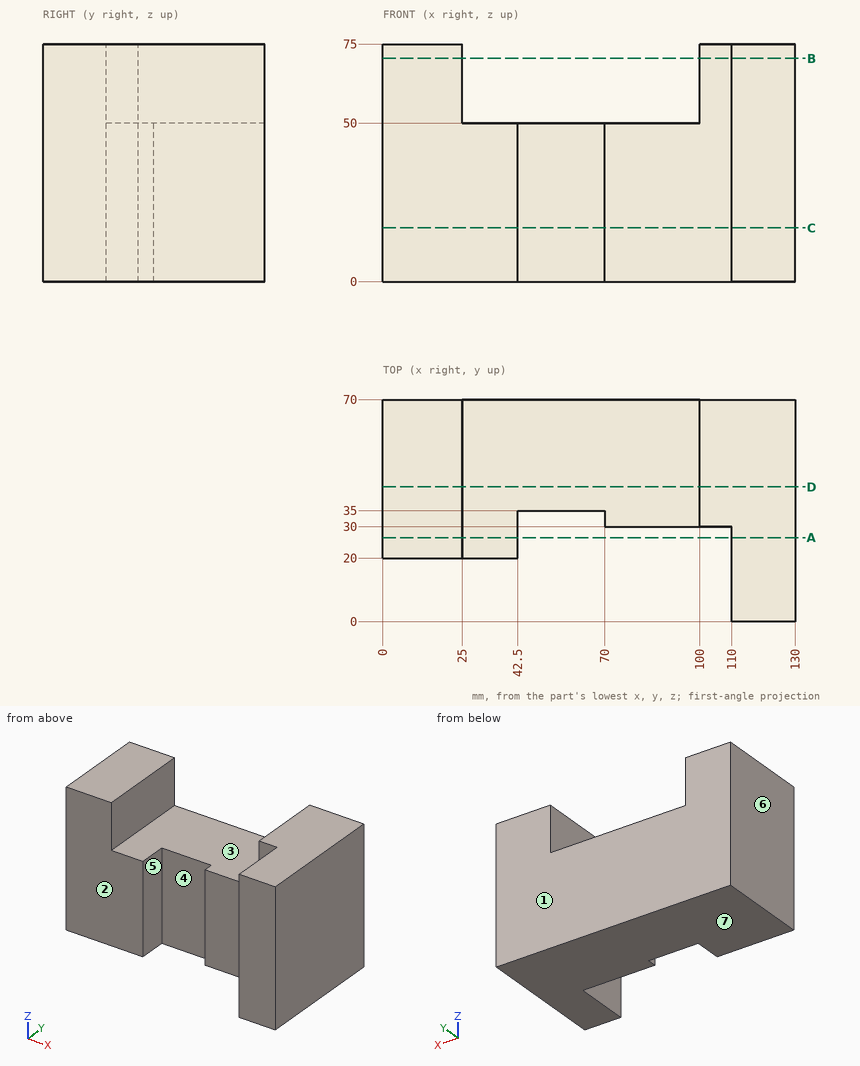
Could you check a few things on this drawing? It's one solid part, dimensions in mm from its lowest x, y, z. A direction names the side the tool comes from. Give positions to 0.01 mm unless a question says otherwise; leave off trailing zeros. Order: outer loops, then holes, each group sorted by start corner. A loop starts at its lowest first (then second) coordinate and runs counter-clockwise, first axis right, second up. Notation, with made-up numbers: M -0.75,60.5 L 51.25,60.5 A22 cw 51.25,84.5 Z; hole C 12.5,-11.75 d8. An arc over 180 degrees is marked long. Use one line per item in the form item = value. Start each with the question number.
Item 1: If we section it at B-B (z = 70.5): Write out the boundary of the cut face in (x, y).
Item 2: We'd pull the mould along X, two halves only. Please class the marked faces 5, 6 and 7: +X half, -X half, draft (parallel to the pull), parting line (faces both ways), or undercut.
Item 3: If we section it at C-C (z = 17): Write out the boundary of the cut face in (x, y), then the cut area to 3 significant figures.
Item 4: If we section it at A-A (y = 26.5): Write out the boundary of the cut face in (x, z), then the cut area to 3 significant figures.
Item 5: For the marked faces 1, 2, 3 and 4, which set-ups out of +Z, -Z, +X, -X, +Y, -Y let a thin tool reach every point of the face, with its end or its side?
Item 6: If I drill on line 1 along X through (y, z) = (22.5, 7.5); line 2 along X through (y, z) = (31, 70); line 3 along Y through (x, z) = (100.5, 30), over which ranges is the centre line in solid material (lowest first)?
Item 7: If we section it at D-D (y = 42.5): Write out the boundary of the cut face in (x, z), then the cut area to 4 significant figures.
Item 8: Will these pins go through, and if not, where does the flat tip stop? pin 1 Ø13 at (x, z) = (26.5, 34.5) entering from -Y; pin 2 Ø6 at (x, z) = (54.5, 21.5) entering from -Y; pin 3 Ø25 at (x, y) = (62, 38.5) entering from +Z.
Outcome:
q1.outline = M 0,20 L 25,20 L 25,70 L 0,70 Z; M 100,30 L 110,30 L 110,0 L 130,0 L 130,70 L 100,70 Z
q2.face_5 = undercut
q2.face_6 = -X half
q2.face_7 = draft
q3.outline = M 0,20 L 42.5,20 L 42.5,35 L 70,35 L 70,30 L 110,30 L 110,0 L 130,0 L 130,70 L 0,70 Z
q3.area = 6,090 mm2
q4.outline = M 0,0 L 42.5,0 L 42.5,50 L 25,50 L 25,75 L 0,75 Z; M 110,0 L 130,0 L 130,75 L 110,75 Z
q4.area = 4,250 mm2
q5.face_1 = +Z, -Z, +X, -X, +Y
q5.face_2 = +Z, -Z, -X, -Y
q5.face_3 = +Z, +Y, -Y
q5.face_4 = +Z, -Z, -Y
q6.line_1 = 0 to 42.5, 110 to 130
q6.line_2 = 0 to 25, 100 to 130
q6.line_3 = 30 to 70
q7.outline = M 0,0 L 130,0 L 130,75 L 100,75 L 100,50 L 25,50 L 25,75 L 0,75 Z
q7.area = 7,875 mm2
q8.pin_1 = 20
q8.pin_2 = 35
q8.pin_3 = 50
